Part print with two shaded views. Sizes in mm from the minimum x, y, z corner. A direction names the side the tool comes from. Give positions to 0.01 mm unless a question says otherwise; leave off trailing zeros. Write each loop counter-clockwise with the first axis right and the second up, starting at its lowest first coordinate (ties: lowest second). Pieces come first, ordered by that corner, then holes.
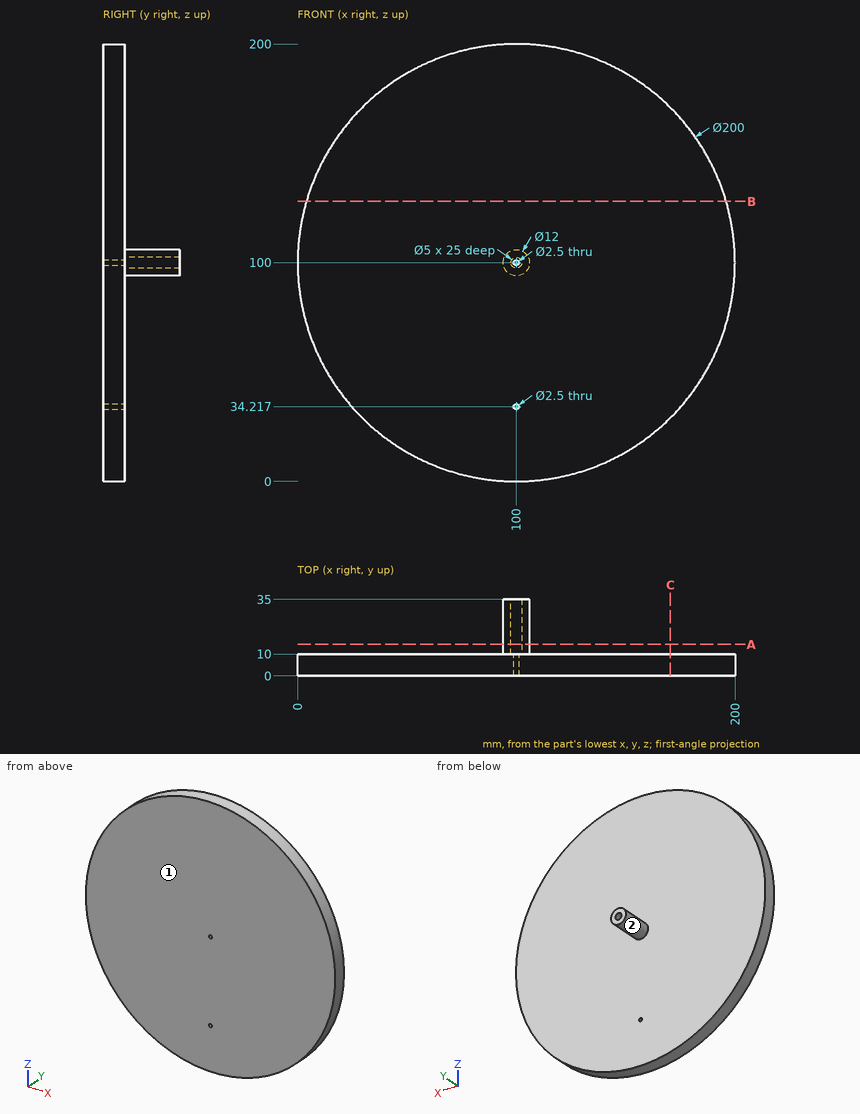
1) Pin check, flat tips, straight feed: pin 1 Ø3 at (x, z) = (100, 34.22) entering from -Y; pin 2 Ø1 at (x, z) = (96.5, 122) entering from +Y; pin 3 Ø2 at (x, y) = (101, 22.5) entering from -Z; pin 4 Ø10 at (y, z) = (15.5, 23.5) entering from -X. Stop position of each tip, or through.
Answers follow:
pin 1: stops at y = 0
pin 2: stops at y = 10
pin 3: stops at z = 94
pin 4: passes through
2) Saw through at C-C, the plane x = 170.5. Write the cut outline in (y, z).
Answers follow:
outline: (0, 29.08) - (10, 29.08) - (10, 170.92) - (0, 170.92) - close
3) Saw through at B-B, the plane z = 128. Write the cut outline in (x, y), then the cut area to 3 significant figures.
Answers follow:
outline: (4, 0) - (196, 0) - (196, 10) - (4, 10) - close
area: 1,920 mm2
4) Wall check: L1, parallel to Z at x = 100, y = 4.5; L2, parallel to Y at x = 149, z = 125; L3, parallel to X at y = 22.5, z = 98.5. Give the ranges that are in metal, low to high.
Answers follow:
L1: z = 0 to 32.97, 35.47 to 98.75, 101.25 to 200
L2: y = 0 to 10
L3: x = 94.19 to 98, 102 to 105.81
5) Saw through at A-A, the plane y = 14.5. Write the cut outline in (x, z).
Answers follow:
outline: circle Ø12 at (100, 100); hole circle Ø5 at (100, 100)
6) 3-axis set-ups, long thin cutter, end or side, ignore diameter. For the marked faces 1 and 2: which of +Z, -Z, +X, -X, +Y, -Y reach the whole face in a straight line?
Answers follow:
face 1: +Z, -Z, +X, -X, -Y
face 2: +Y
